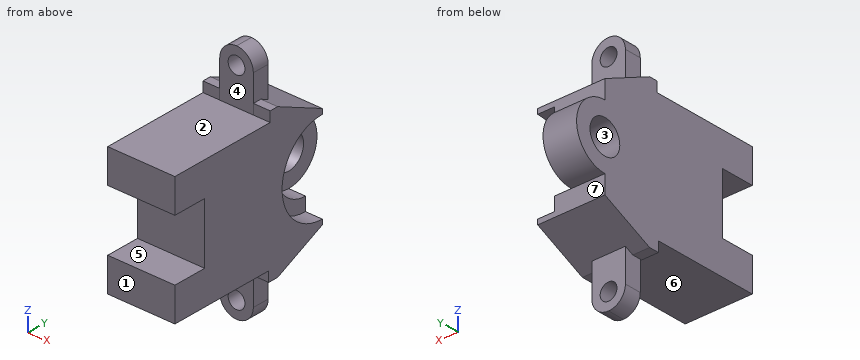
from build123d import *

# Parameters (mm, degrees)
BOSS_EXTRUDE1_DEPTH      = 40
BOSS_EXTRUDE2_DEPTH      = 110
BOSS_EXTRUDE2_DEPTH_BACK = 31
SKETCH11_R               = 5
CUT_EXTRUDE11_DEPTH      = 30
SKETCH12_R               = 5
CUT_EXTRUDE15_DEPTH      = 84
SKETCH5_W                = 36
SKETCH5_H                = 20
CUT_EXTRUDE3_DEPTH       = 43
BOSS_EXTRUDE6_DEPTH      = 40
CUT_EXTRUDE4_START       = -10
SKETCH6_R                = 27
CUT_EXTRUDE4_DEPTH       = 10
CUT_EXTRUDE7_START       = -10
CUT_EXTRUDE7_DEPTH       = 10
CUT_EXTRUDE8_START       = -20
CUT_EXTRUDE8_DEPTH       = 20
SKETCH10_R               = 10
CUT_EXTRUDE9_DEPTH       = 20


# Read off the part's stored shape, not the designer's step: Boss-Extrude6
with BuildPart() as part:
    # Sketch1 → Boss-Extrude1 (new body)
    with BuildSketch(Plane(origin=(0, 0, 0), x_dir=(0, 0, -1), z_dir=(1, 0, 0))):
        Polygon((-38.7187028, -36.676276186), (37.2812972, -36.676276186), (37.2812972, 26.323723814), (43.2812972, 26.323723814), (43.2812972, 32.323723814), (29.2812972, 62.323723814), (-30.7187028, 62.323723814), (-44.7187028, 32.323723814), (-44.7187028, 27.323723814), (-38.7187028, 27.323723814), align=None)
    extrude(amount=BOSS_EXTRUDE1_DEPTH)

    # 3DSketch1 → Boss-Extrude2 (add, two sides: drawn at the far end of the back side and taken through both)
    with BuildSketch(Plane(origin=(30, 37.289381844, 39.546748703), x_dir=(-0.8944271909999159, -0.44721359549995804, 0), z_dir=(0, 0, -1)).offset(-BOSS_EXTRUDE2_DEPTH_BACK)):
        Polygon((0, 0), (17.88854382, 8.94427191), (22.360679775, 0), (4.472135955, -8.94427191), align=None)
    extrude(amount=BOSS_EXTRUDE2_DEPTH + BOSS_EXTRUDE2_DEPTH_BACK)

    # Sketch11 → Cut-Extrude11 (cut)
    with BuildSketch(Plane(origin=(0, 37.289381844, 0), x_dir=(1, 0, 0), z_dir=(0, 1, 0))):
        with BuildLine():
            Line((20, 70.453251297), (10, 70.453251297))
            Line((10, 70.453251297), (10, 60.453251297))
            ThreePointArc((10, 60.453251297), (12.928932188, 67.524319109), (20, 70.453251297))
        make_face()
        with BuildLine():
            Line((30, 70.453251297), (20, 70.453251297))
            ThreePointArc((20, 70.453251297), (27.071067812, 67.524319109), (30, 60.453251297))
            Line((30, 60.453251297), (30, 70.453251297))
        make_face()
        with Locations(Location((20, 60.453251297, 0), (0, 0, 270))):
            Circle(SKETCH11_R)
    extrude(amount=-CUT_EXTRUDE11_DEPTH, mode=Mode.SUBTRACT)

    # Sketch12 → Cut-Extrude15 (cut)
    with BuildSketch(Plane(origin=(0, 0, 0), x_dir=(1, 0, 0), z_dir=(0, 1, 0))):
        with BuildLine():
            Line((10, -70.546748703), (20, -70.546748703))
            ThreePointArc((20, -70.546748703), (12.928932188, -67.617816515), (10, -60.546748703))
            Line((10, -60.546748703), (10, -70.546748703))
        make_face()
        with BuildLine():
            Line((20, -70.546748703), (30, -70.546748703))
            Line((30, -70.546748703), (30, -60.546748703))
            ThreePointArc((30, -60.546748703), (27.071067812, -67.617816515), (20, -70.546748703))
        make_face()
        with Locations(Location((20, -60.546748703, 0), (0, 0, 90))):
            Circle(SKETCH12_R)
    extrude(amount=CUT_EXTRUDE15_DEPTH, mode=Mode.SUBTRACT)

    # Sketch5 → Cut-Extrude3 (cut)
    with BuildSketch(Plane(origin=(40, 0, 0), x_dir=(0, 0, -1), z_dir=(1, 0, 0))):
        with Locations((-0.7187028, -26.676276186)):
            Rectangle(SKETCH5_W, SKETCH5_H)
    extrude(amount=-CUT_EXTRUDE3_DEPTH, mode=Mode.SUBTRACT)

    # Boss-Extrude6 outline → Boss-Extrude6 (add)
    with BuildSketch(Plane.YZ):
        with BuildLine():
            ThreePointArc((62.323723814, -26.2812972), (89.323723814, 0.7187028), (62.323723814, 27.7187028))
            Line((62.323723814, 27.7187028), (62.323723814, -26.2812972))
        make_face()
    extrude(amount=BOSS_EXTRUDE6_DEPTH)

    # Sketch6 → Cut-Extrude4 (cut)
    with BuildSketch(Plane(origin=(40, 0, 0), x_dir=(0, 0, -1), z_dir=(1, 0, 0)).offset(CUT_EXTRUDE4_START)):
        with Locations((-0.7187028, 62.323723814)):
            Circle(SKETCH6_R)
    extrude(amount=CUT_EXTRUDE4_DEPTH, mode=Mode.SUBTRACT)

    # Sketch8 → Cut-Extrude7 (cut)
    with BuildSketch(Plane(origin=(30, 0, 0), x_dir=(0, 0, -1), z_dir=(1, 0, 0)).offset(CUT_EXTRUDE7_START)):
        with BuildLine():
            Line((-27.7187028, 62.323723814), (-19.7187028, 62.323723814))
            ThreePointArc((-19.7187028, 62.323723814), (-0.7187028, 43.323723814), (18.2812972, 62.323723814))
            Line((18.2812972, 62.323723814), (26.2812972, 62.323723814))
            ThreePointArc((26.2812972, 62.323723814), (-0.7187028, 89.323723814), (-27.7187028, 62.323723814))
        make_face()
    extrude(amount=CUT_EXTRUDE7_DEPTH, mode=Mode.SUBTRACT)

    # Sketch9 → Cut-Extrude8 (cut)
    with BuildSketch(Plane(origin=(20, 0, 0), x_dir=(0, 0, -1), z_dir=(1, 0, 0)).offset(CUT_EXTRUDE8_START)):
        with BuildLine():
            Line((-27.7187028, 62.323723814), (-19.7187028, 62.323723814))
            ThreePointArc((-19.7187028, 62.323723814), (-0.7187028, 81.323723814), (18.2812972, 62.323723814))
            Line((18.2812972, 62.323723814), (26.2812972, 62.323723814))
            ThreePointArc((26.2812972, 62.323723814), (-0.7187028, 89.323723814), (-27.7187028, 62.323723814))
        make_face()
    extrude(amount=CUT_EXTRUDE8_DEPTH, mode=Mode.SUBTRACT)

    # Sketch10 → Cut-Extrude9 (cut)
    with BuildSketch(Plane(origin=(20, 0, 0), x_dir=(0, 0, -1), z_dir=(1, 0, 0))):
        with Locations((-0.7187028, 62.323723814)):
            Circle(SKETCH10_R)
    extrude(amount=-CUT_EXTRUDE9_DEPTH, mode=Mode.SUBTRACT)


solid = part.part
Part model, mm, in its own coordinate system. Face numbers are marked on the shaded views. A direction names the side the tool comes from. Coordinates: 2 decimals unless noted, no trailing zeros. Order: outer loops, then holes, each group sorted by start corner. A loop starts at its lowest first (then second) coordinate and runs counter-clockwise, first axis right, second up. Notation, with made-up numbers: M 35,82 L 51,82 A24 cw 51,95 Z; hole C 0,29 d9. An arc over 180 degrees is marked long. Use a Markdown table: item, result.
(1) Cut at A-A on x = 17.5. State how many separate pieces and enclosed holes the cut face has, then the cut area to 3 significant figures.
A:
| item | result |
|---|---|
| separate pieces | 3 |
| enclosed holes | 1 |
| area | 7,430 mm^2 |
(2) Tool access for the marked faces 4, 5, 6 and 7: list every direction of +Z, -Z, +X, -X, +Y, -Y with a clear straight run to the whole face (end or side of a thin tool).
A:
| item | result |
|---|---|
| face 4 | +Z, +X, -X, -Y |
| face 5 | +X, -X, -Y |
| face 6 | -Z, +X, -X, -Y |
| face 7 | -Z, +X, -X, +Y |
(3) Probe L1, parallel to Z at x = 27, y = -26; L2, parallel to Z at x = 21, y = -15.5; L3, parallel to Y at x = 12, z = -49. List the from-to ranges inside material, lowest first.
A:
| item | result |
|---|---|
| L1 | z = -37.28 to -17.28, 18.72 to 38.72 |
| L2 | z = -37.28 to 38.72 |
| L3 | y = 27.29 to 37.29 |
(4) Cut at D-D on x = 8. Write the cut outline in (y, z).
A:
| item | result |
|---|---|
| outline | M -36.68,-37.28 L 26.32,-37.28 L 26.32,-43.28 L 32.32,-43.28 L 62.32,-29.28 L 62.32,-18.28 A19 ccw 62.32,19.72 L 62.32,30.72 L 32.32,44.72 L 27.32,44.72 L 27.32,38.72 L -36.68,38.72 L -36.68,18.72 L -16.68,18.72 L -16.68,-17.28 L -36.68,-17.28 Z; hole C 62.32,0.72 d20 |
(5) Pull direction Z, two halves, no side cores. Call the marked faces 1, 2 and 3: released by +Z, released by -Z, zero draft, split by the parting line, or undercut.
A:
| item | result |
|---|---|
| face 1 | zero draft |
| face 2 | released by +Z |
| face 3 | undercut |
(6) Cut at C-C on y = 56.5. Write the cut outline in (x, z).
A:
| item | result |
|---|---|
| outline | M 0,-32 L 40,-32 L 40,-25.65 L 30,-25.65 L 30,-17.37 L 20,-17.37 L 20,-7.41 L 0,-7.41 Z; M 0,8.85 L 20,8.85 L 20,18.8 L 30,18.8 L 30,27.08 L 40,27.08 L 40,33.44 L 0,33.44 Z |
(7) Cut at B-B on z = 7.5. Write the cut outline in (x, y), then the cut area to 3 significant figures.
A:
| item | result |
|---|---|
| outline | M 0,-16.68 L 40,-16.68 L 40,36.19 L 30,36.19 L 30,44.58 L 20,44.58 L 20,54.97 L 0,54.97 Z; M 0,69.67 L 20,69.67 L 20,80.07 L 0,80.07 Z |
| area | 2,780 mm^2 |
(8) Flat gauge pins, fed straight in: pin 1 (5.5 mm diameter, centred on x = 29.5, z = -22.5, fed in from +Y); pin 2 (1.5 mm diameter, centred on y = 67, z = 12.5, fed in from +X); pin 3 (1 mm diameter, centred on x = 25, y = -7, fed in from -Z); pin 4 (8 mm diameter, centred on x = 20, z = 60.55, fed in from +Y). Where does each tip first touch, or does it go through?
A:
| item | result |
|---|---|
| pin 1 | stops at y = 62.32 |
| pin 2 | stops at x = 20 |
| pin 3 | stops at z = -37.28 |
| pin 4 | passes through |
